Can you work these out from the model? Positions are in its coordinate system, mm. A direction names the side the tool comes from. Give positions to 0.01 mm unless a question says otherwise; leave off trailing zeros. Order: outer loops, then holes, each group sorted by start corner. A loop starts at its lowest first (then second) coordinate and runs counter-clockwise, first axis right, second up. Notation, with made-up numbers: (85.25, 83) - (100.25, 83) arc R13 ccw to (100.25, 87) - close; hole circle Ø10 at (57, -10.75). An arc over 180 degrees is marked (long way). Return JSON: item names as keys, results as strings.
```python
from build123d import *

# Parameters (mm, degrees)
F0_W     = 12.7
F0_H     = 3.81
F1_DEPTH = 3.81
F2_R     = 2.2225
F3_DEPTH = 31.75


with BuildPart() as f1:
    # F0 (on Top) → F1 (new body)
    with BuildSketch(Plane.XY):
        Polygon((3.175, 57.15), (-3.175, 57.15), (-3.175, 43.33875), (-3.175, 39.52875), (-3.175, 15.71625), (-3.175, 11.90625), (-3.175, -11.90625), (-3.175, -15.71625), (-3.175, -39.52875), (-3.175, -43.33875), (-3.175, -57.15), (3.175, -57.15), (3.175, -53.34), (3.175, -29.5275), (3.175, -25.7175), (3.175, -1.905), (3.175, 1.905), (3.175, 25.7175), (3.175, 29.5275), (3.175, 53.34), align=None)
        with Locations((-9.525, -41.43375)):
            Rectangle(F0_W, F0_H)
        with Locations((9.525, 0)):
            Rectangle(F0_W, F0_H)
        with Locations((9.525, 55.245)):
            Rectangle(F0_W, F0_H)
        with Locations((-9.525, -13.81125)):
            Rectangle(F0_W, F0_H)
        with Locations((9.525, 27.6225)):
            Rectangle(F0_W, F0_H)
        with Locations((9.525, -55.245)):
            Rectangle(F0_W, F0_H)
        with Locations((-9.525, 13.81125)):
            Rectangle(F0_W, F0_H)
        with Locations((9.525, -27.6225)):
            Rectangle(F0_W, F0_H)
        with Locations((-9.525, 41.43375)):
            Rectangle(F0_W, F0_H)
    extrude(amount=F1_DEPTH)

    # F2 (on face) → F3 (join)
    with BuildSketch(Plane.XY.offset(3.81)):
        Circle(F2_R)
        with Locations((0, 17.78)):
            Circle(F2_R)
        with Locations((0, 35.56)):
            Circle(F2_R)
        with Locations((0, 53.34)):
            Circle(F2_R)
        with Locations((0, -17.78)):
            Circle(F2_R)
        with Locations((0, -35.56)):
            Circle(F2_R)
        with Locations((0, -53.34)):
            Circle(F2_R)
    extrude(amount=F3_DEPTH)


solid = f1.part
```
1. If I drill on L1, parallel to Y at x = -9.5, z = 3.5; L2, parallel to Z at x = -11.5, y = -13.5; L3, parallel to X at y = -18.5, z = 3 (3 decimals), over which ranges is the centre line in solid material (lowest first)? Write a range as [from, to].
Checks:
{"L1": "[-43.34, -39.53], [-15.72, -11.91], [11.91, 15.72], [39.53, 43.34]", "L2": "[0, 3.81]", "L3": "[-3.175, 3.175]"}
2. Suppose I cut it at C-C (x = 12). State how many separate pieces and enclosed holes the cut face has, plus the area to 3 significant figures.
Checks:
{"separate pieces": "5", "enclosed holes": "0", "area": "72.6 mm^2"}
3. On a 3-axis mill with a long thin cutter (end or side, diameter ignored), from which of +Z, -Z, +X, -X, +Y, -Y can I reach the whole of each face in a straight line? I mean faces 4 (the face through (0, 0, 35.56)), 5 (the face through (3.175, 14, 2)), 6 (the face through (-15.875, -14, 2)), 7 (the face through (-0.289, 55.544, 19.463)), 8 (the face through (-3.175, 0, 2)). Say none if no direction works.
Checks:
{"face 4": "+Z, +X, -X, +Y, -Y", "face 5": "+Z, -Z, +X", "face 6": "+Z, -Z, -X, +Y, -Y", "face 7": "+Z", "face 8": "+Z, -Z, -X"}
4. Thinking about a two-plate mould opening in Y: for faces 1 (the face through (-10, -43.339, 2)), 2 (the face through (-10, 15.716, 2)), 3 (the face through (0, 18, 35.56)), which applies, +Y half, -Y half, draft (parallel to the pull), parting line (faces both ways), or undercut?
Checks:
{"face 1": "-Y half", "face 2": "undercut", "face 3": "draft"}
5. Suppose I cut it at A-A (x = -12). List the corners of the cut face in (y, z) for me.
Checks:
{"outline": "(-43.34, 0) - (-39.53, 0) - (-39.53, 3.81) - (-43.34, 3.81) - close; (-15.72, 0) - (-11.91, 0) - (-11.91, 3.81) - (-15.72, 3.81) - close; (11.91, 0) - (15.72, 0) - (15.72, 3.81) - (11.91, 3.81) - close; (39.53, 0) - (43.34, 0) - (43.34, 3.81) - (39.53, 3.81) - close"}
6. Suppose I cut it at D-D (y = 35.56). List the corners of the cut face in (x, z) for me (1 decimal), plus the area to 3 significant figures.
Checks:
{"outline": "(-3.2, 0) - (3.2, 0) - (3.2, 3.8) - (2.2, 3.8) - (2.2, 35.6) - (-2.2, 35.6) - (-2.2, 3.8) - (-3.2, 3.8) - close", "area": "165 mm^2"}
7. Suppose I cut it at B-B (z = 10). List the corners of the cut face in (x, y) for me (1 decimal).
Checks:
{"outline": "circle Ø4.4 at (0, -53.3); circle Ø4.4 at (0, -35.6); circle Ø4.4 at (0, -17.8); circle Ø4.4 at (0, 0); circle Ø4.4 at (0, 17.8); circle Ø4.4 at (0, 35.6); circle Ø4.4 at (0, 53.3)"}
8. For pin 1 Ø1.9 at (y, z) = (-8, 2.5) entering from +X (3 decimals); pin 2 Ø1.9 at (y, z) = (50.5, 1.5) entering from -X (3 decimals); pin 3 Ø2 at (x, y) = (-12, -16.5) entering from +Z; pin 4 Ø1.5 at (x, y) = (1.5, -23) entering from -Z, each with a flat end and sliding along its axis, tell me the tip position at first contact or that it passes through.
Checks:
{"pin 1": "x = 3.175", "pin 2": "x = -3.175", "pin 3": "z = 3.81", "pin 4": "z = 0"}
